Verification items for this drawing (mm, ordinates from the low corner). A direction names the side the tool comes from. Coordinates: 2 decimals unless noted, no trailing zeros. Loops run counter-clockwise (first coordinate to the right, second up) from the corner with the lowest first, then second, coordinate; pieces in that order, holes last. Notation, with made-up numbers: (17, 10.5) - (49, 10.5) arc R33 cw to (49, 44.5) - close; hole circle Ø2 at (-33.5, 12). An arc over 180 degrees is marked (long way). One line per item, written item: value. Start each with the question number.
(1) Draft check along X on the marked faces 1, 2, 3 and 4. Enter one of: +X half, -X half, draft (parallel to the pull), parting line (faces both ways), or undercut.
(2) Section check C-C (x = 27.5). Record the boundary of the cut face in (y, z), plus the area to 3 significant figures.
(3) Set-up check for the marked faces 5 and 6: record each of +Z, -Z, +X, -X, +Y, -Y from which the full face is reachable in a straight line by a thin tool's end or side.
(4) Gauge pin test, flat ends, axial feed: P1, Ø1.5, axis at x = 32.5, z = 23, coming from the -Y side (1 decimal); P2, Ø1.5, axis at x = 26.5, z = 28.5, coming from the +Y side (3 decimals); P3, Ø8, axis at x = 24, z = 30.5, coming from the -Y side. Record the tip position at first contact, or that the pin passes through.
(5) Section check A-A (y = 35). Record the boundary of the cut face in (x, z), plus the area to 3 significant figures.
(6) Section check B-B (z = 12.5). Record the boundary of the cut face in (x, y), plus the area to 3 significant figures.
(7) Thickness scan on probe 1 along Z at (x, y) = (17, 64.5); probe 2 along Y at (x, z) = (10, 17.5); probe 3 along Y at (x, z) = (33, 10.5). Record the ranges inside material, lowest first. Write a range as [from, to].
(8) Section check D-D (x = 48). Record the boundary of the cut face in (y, z).
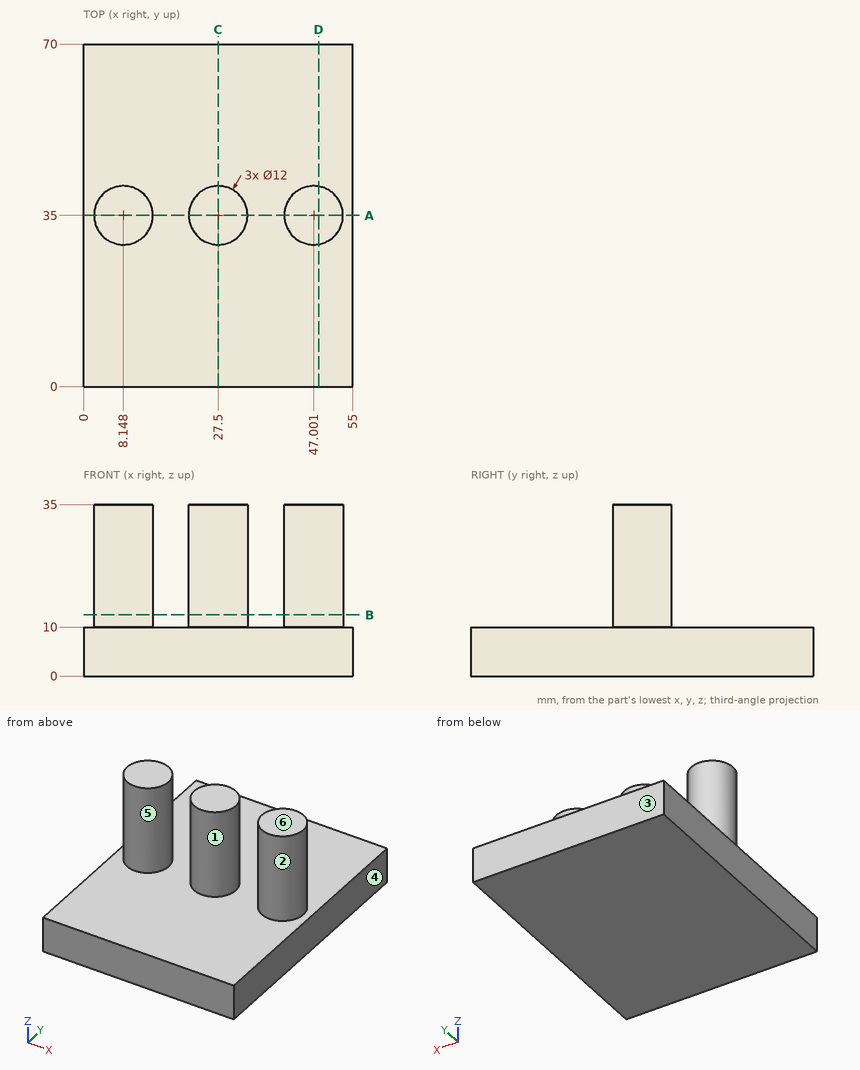
Responses:
1. face 1: undercut
1. face 2: undercut
1. face 3: draft
1. face 4: +X half
2. outline: (0, 0) - (70, 0) - (70, 10) - (41, 10) - (41, 35) - (29, 35) - (29, 10) - (0, 10) - close
2. area: 1,000 mm²
3. face 5: +Z
3. face 6: +Z, +X, -X, +Y, -Y
4. P1: stops at y = 30.8
4. P2: stops at y = 40.995
4. P3: stops at y = 29
5. outline: (0, 0) - (55, 0) - (55, 10) - (53, 10) - (53, 35) - (41, 35) - (41, 10) - (33.5, 10) - (33.5, 35) - (21.5, 35) - (21.5, 10) - (14.15, 10) - (14.15, 35) - (2.15, 35) - (2.15, 10) - (0, 10) - close
5. area: 1,450 mm²
6. outline: circle Ø12 at (8.15, 35); circle Ø12 at (27.5, 35); circle Ø12 at (47, 35)
6. area: 339 mm²
7. probe 1: z = [0, 10]
7. probe 2: y = [29.29, 40.71]
7. probe 3: y = [32.6, 37.4]
8. outline: (0, 0) - (70, 0) - (70, 10) - (40.92, 10) - (40.92, 35) - (29.08, 35) - (29.08, 10) - (0, 10) - close
